The listing builds one solid part. Answer for the finished solid, in the listing's coordinates (mm). Face numbers are marked on the shaded views. A direction names the side the tool comes from. Round coordinates to 2 decimals unless told otherwise and drop trailing zeros. Write each loop counter-clockwise with the first axis right and the second up, starting at its lowest first coordinate (ties: lowest second). Pieces come first, ordered by that corner, then holes.
(1) For the marked faces 1 and 2, determine the directions among +Z, -Z, +X, -X, +Y, -Y from which every point of the face is accessible in a straight line to the end or side of a thin tool.
(2) The mould has two halves that part along Y. Classify the marked faces 3, 4, 5 and 6: +Y half, -Y half, draft (parallel to the pull), parting line (faces both ways), or undercut.
(3) Each of these flat-tipped pins is pushed along its axis until it touches: pin 1 Ø0.9 at (x, y) = (-99, 20) entering from -Z; pin 2 Ø3 at (y, z) = (4.5, 0.5) entering from -X; pin 3 Ø0.9 at (x, y) = (-97.5, 14.5) entering from +Z; pin 4 Ø5 at (y, z) = (17, 0.5) entering from -X. Where does it stop, or does it pass through?
(4) Find the intervals of material crossed by probe 1 along X at (y, z) = (14, -14); probe 2 along Y at (x, z) = (7, 15.5); probe 3 along Z at (x, y) = (6.5, 28), in increasing order.
(5) A cutting plane is placed at A-A, the plane z = 17.5. Give the vertices of the cut face in (x, y), and give its area (3 significant figures).
(6) A cutting plane is placed at C-C, the plane y = 6. Give the number of separate pieces and of enclosed holes in the cut face, and give its area (3 significant figures).
from build123d import *

# Parameters (mm, degrees)
SKETCH1_W           = 192
SKETCH1_H           = 42.3
BOSS_EXTRUDE1_DEPTH = 2
SKETCH2_W           = 176
SKETCH2_H           = 2
BOSS_EXTRUDE2_DEPTH = 30.35
SKETCH3_W           = 192
SKETCH3_H           = 42.3
BOSS_EXTRUDE3_DEPTH = 2
FILLET1_R           = 12
FILLET2_R           = 12
FILLET3_R           = 12
FILLET4_R           = 12
CUT_EXTRUDE1_DEPTH  = 2
CUT_EXTRUDE2_DEPTH  = 2
SKETCH6_R           = 4
BOSS_EXTRUDE5_DEPTH = 6
SKETCH7_R           = 2.25
CUT_EXTRUDE3_DEPTH  = 10
SKETCH8_W           = 1.5
SKETCH8_H           = 9.217326718
CUT_EXTRUDE4_DEPTH  = 6
SKETCH10_R          = 1.5
CUT_EXTRUDE9_DEPTH  = 6
FILLET5_R           = 2
FILLET6_R           = 2
FILLET9_R           = 2
FILLET10_R          = 2
FILLET11_R          = 2
FILLET14_R          = 1
FILLET15_R          = 1
SKETCH11_R          = 2.5
CUT_EXTRUDE11_DEPTH = 1
SKETCH12_R          = 4.5
CUT_EXTRUDE12_DEPTH = 1
SKETCH13_R          = 2.5
CUT_EXTRUDE14_DEPTH = 10
SKETCH14_W          = 29
SKETCH14_H          = 29
CUT_EXTRUDE15_DEPTH = 2
SKETCH15_R          = 4.5
CUT_EXTRUDE16_DEPTH = 1
FILLET16_R          = 0.5
FILLET17_R          = 0.5
SKETCH16_W          = 8
SKETCH16_H          = 30.35
CUT_EXTRUDE17_DEPTH = 80
FILLET18_R          = 2
FILLET19_R          = 2


with BuildPart() as part:
    # Sketch1 → Boss-Extrude1 (new body)
    with BuildSketch(Plane(origin=(0, 0, 0), x_dir=(1, 0, 0), z_dir=(0, 1, 0))):
        Rectangle(SKETCH1_W, SKETCH1_H)
    extrude(amount=BOSS_EXTRUDE1_DEPTH)

    # Sketch2 → Boss-Extrude2 (add)
    with BuildSketch(Plane(origin=(0, 2, 0), x_dir=(1, 0, 0), z_dir=(0, 1, 0))):
        Polygon((-96, 21.15), (-96, -21.15), (-88, -21.15), (-88, 19.15), (-88, 21.15), align=None)
        with Locations((0, 20.15)):
            Rectangle(SKETCH2_W, SKETCH2_H)
        Polygon((88, 19.15), (88, -21.15), (96, -21.15), (96, 21.15), (88, 21.15), align=None)
    extrude(amount=BOSS_EXTRUDE2_DEPTH)

    # Sketch3 → Boss-Extrude3 (add)
    with BuildSketch(Plane(origin=(0, 32.35, 0), x_dir=(1, 0, 0), z_dir=(0, 1, 0))):
        Rectangle(SKETCH3_W, SKETCH3_H)
    extrude(amount=BOSS_EXTRUDE3_DEPTH)

    # Fillet1
    fillet1_edges = [part.edges().sort_by_distance(p)[0] for p in [
        (-88, 32.35, 1),
    ]]
    fillet(fillet1_edges, radius=FILLET1_R)

    # Fillet2
    fillet2_edges = [part.edges().sort_by_distance(p)[0] for p in [
        (-88, 2, 1),
    ]]
    fillet(fillet2_edges, radius=FILLET2_R)

    # Fillet3
    fillet3_edges = [part.edges().sort_by_distance(p)[0] for p in [
        (88, 32.35, 1),
    ]]
    fillet(fillet3_edges, radius=FILLET3_R)

    # Fillet4
    fillet4_edges = [part.edges().sort_by_distance(p)[0] for p in [
        (88, 2, 1),
    ]]
    fillet(fillet4_edges, radius=FILLET4_R)

    # Sketch4 → Cut-Extrude1 (cut)
    with BuildSketch(Plane.XY.offset(-19.15)):
        with BuildLine():
            Line((-76, 32.35), (-88, 20.35))
            ThreePointArc((-88, 20.35), (-84.485281374, 28.835281374), (-76, 32.35))
        make_face()
        with BuildLine():
            Line((-88, 14), (-76, 2))
            ThreePointArc((-76, 2), (-84.485281374, 5.514718626), (-88, 14))
        make_face()
        Polygon((-76, 32.35), (-88, 20.35), (-88, 14), (-76, 2), (-26, 2), (-26, 32.35), align=None)
    extrude(amount=-CUT_EXTRUDE1_DEPTH, mode=Mode.SUBTRACT)

    # Sketch5 → Cut-Extrude2 (cut)
    with BuildSketch(Plane.XY.offset(-19.15)):
        Polygon((88, 20.35), (76, 32.35), (26, 32.35), (26, 2), (76, 2), (88, 14), align=None)
        with BuildLine():
            Line((88, 20.35), (76, 32.35))
            ThreePointArc((76, 32.35), (84.485281374, 28.835281374), (88, 20.35))
        make_face()
        with BuildLine():
            Line((76, 2), (88, 14))
            ThreePointArc((88, 14), (84.485281374, 5.514718626), (76, 2))
        make_face()
    extrude(amount=-CUT_EXTRUDE2_DEPTH, mode=Mode.SUBTRACT)

    # Sketch6 → Boss-Extrude5 (add)
    with BuildSketch(Plane.ZY.offset(96)):
        with Locations(Location((0, 17.175, 0), (0, 0, 180))):
            Circle(SKETCH6_R)
    extrude(amount=BOSS_EXTRUDE5_DEPTH)

    # Sketch7 → Cut-Extrude3 (cut)
    with BuildSketch(Plane.ZY.offset(102)):
        with Locations((0, 17.175)):
            Circle(SKETCH7_R)
    extrude(amount=-CUT_EXTRUDE3_DEPTH, mode=Mode.SUBTRACT)

    # Sketch8 → Cut-Extrude4 (cut)
    with BuildSketch(Plane.ZY.offset(102)):
        with Locations((0, 17.175)):
            Rectangle(SKETCH8_W, SKETCH8_H)
    extrude(amount=-CUT_EXTRUDE4_DEPTH, mode=Mode.SUBTRACT)

    # Sketch10 → Cut-Extrude9 (cut)
    with BuildSketch(Plane.XZ):
        with Locations(Location((-18.002866527, -3.655663128, 0), (0, 0, 270))):
            Circle(SKETCH10_R)
        with Locations(Location((17.997133473, -3.655663128, 0), (0, 0, 270))):
            Circle(SKETCH10_R)
    extrude(amount=-CUT_EXTRUDE9_DEPTH, mode=Mode.SUBTRACT)

    # Fillet5
    fillet5_edges = [part.edges().sort_by_distance(p)[0] for p in [
        (0, 0, -21.15),
    ]]
    fillet(fillet5_edges, radius=FILLET5_R - 0.0001)  # a hair under: the kernel refuses the full size

    # Fillet6
    fillet6_edges = [part.edges().sort_by_distance(p)[0] for p in [
        (0, 34.35, -21.15),
    ]]
    fillet(fillet6_edges, radius=FILLET6_R - 0.0001)  # a hair under: the kernel refuses the full size

    # Fillet9
    fillet9_edges = [part.edges().sort_by_distance(p)[0] for p in [
        (96, 0.585757148, -20.564242852),
        (96, 17.175, -21.15),
        (96, 33.764242852, -20.564242852),
        (96, 34.35, 0.99995),
        (96, 0, 0.99995),
    ]]
    fillet(fillet9_edges, radius=FILLET9_R - 0.0001)  # a hair under: the kernel refuses the full size

    # Fillet10
    fillet10_edges = [part.edges().sort_by_distance(p)[0] for p in [
        (-96, 0, 0.99995),
        (-96, 0.585757148, -20.564242852),
        (-96, 34.35, 0.99995),
        (-96, 17.175, -21.15),
        (-96, 33.764242852, -20.564242852),
    ]]
    fillet(fillet10_edges, radius=FILLET10_R - 0.0001)  # a hair under: the kernel refuses the full size

    # Fillet11
    fillet11_edges = [part.edges().sort_by_distance(p)[0] for p in [
        (96, 17.175, 21.15),
        (95.414242852, 0.585757148, 21.15),
        (95.414242852, 33.764242852, 21.15),
        (0, 34.35, 21.15),
        (-96, 17.175, 21.15),
        (0, 0, 21.15),
        (-95.414242852, 0.585757148, 21.15),
        (-95.414242852, 33.764242852, 21.15),
    ]]
    fillet(fillet11_edges, radius=FILLET11_R - 0.0001)  # a hair under: the kernel refuses the full size

    # Fillet14
    fillet14_edges = [part.edges().sort_by_distance(p)[0] for p in [
        (-102, 17.175, 4),
    ]]
    fillet(fillet14_edges, radius=FILLET14_R)

    # Fillet15
    fillet15_edges = [part.edges().sort_by_distance(p)[0] for p in [
        (-102, 17.175, -4),
    ]]
    fillet(fillet15_edges, radius=FILLET15_R)

    # Sketch11 → Cut-Extrude11 (cut)
    with BuildSketch(Plane(origin=(0, 0, 0), x_dir=(-1, 0, 0), z_dir=(0, -1, 0))):
        with Locations(Location((18.002866527, 3.655663128, 0), (0, 0, 90))):
            Circle(SKETCH11_R)
        with Locations(Location((-17.997133473, 3.655663128, 0), (0, 0, 90))):
            Circle(SKETCH11_R)
    extrude(amount=-CUT_EXTRUDE11_DEPTH, mode=Mode.SUBTRACT)

    # Sketch12 → Cut-Extrude12 (cut)
    with BuildSketch(Plane(origin=(96, 0, 0), x_dir=(0, 0, -1), z_dir=(1, 0, 0))):
        with Locations((0.090844805, 17.432374702)):
            Circle(SKETCH12_R)
    extrude(amount=-CUT_EXTRUDE12_DEPTH, mode=Mode.SUBTRACT)

    # Sketch13 → Cut-Extrude14 (cut)
    with BuildSketch(Plane(origin=(96, 0, 0), x_dir=(0, 0, -1), z_dir=(1, 0, 0))):
        with Locations((0.090844805, 17.432374702)):
            Circle(SKETCH13_R)
    extrude(amount=-CUT_EXTRUDE14_DEPTH, mode=Mode.SUBTRACT)

    # Sketch14 → Cut-Extrude15 (cut)
    with BuildSketch(Plane(origin=(96, 0, 0), x_dir=(0, 0, -1), z_dir=(1, 0, 0))):
        with Locations((0.090844805, 17.432374702)):
            Rectangle(SKETCH14_W, SKETCH14_H)
    extrude(amount=-CUT_EXTRUDE15_DEPTH, mode=Mode.SUBTRACT)

    # Sketch15 → Cut-Extrude16 (cut)
    with BuildSketch(Plane(origin=(94, 0, 0), x_dir=(0, 0, -1), z_dir=(1, 0, 0))):
        with Locations((0.090844805, 17.432374702)):
            Circle(SKETCH15_R)
    extrude(amount=-CUT_EXTRUDE16_DEPTH, mode=Mode.SUBTRACT)

    # Fillet16
    fillet16_edges = [part.edges().sort_by_distance(p)[0] for p in [
        (-102, 18.474038106, 1.837117307),
    ]]
    fillet(fillet16_edges, radius=FILLET16_R)

    # Fillet17
    fillet17_edges = [part.edges().sort_by_distance(p)[0] for p in [
        (-102, 17.175, -2.25),
    ]]
    fillet(fillet17_edges, radius=FILLET17_R)

    # Sketch16 → Cut-Extrude17 (cut)
    with BuildSketch(Plane(origin=(0, 0, -21.15), x_dir=(-1, 0, 0), z_dir=(0, 0, -1))):
        with Locations((-22, 17.175)):
            Rectangle(SKETCH16_W, SKETCH16_H)
        with Locations((22, 17.175)):
            Rectangle(SKETCH16_W, SKETCH16_H)
    extrude(amount=-CUT_EXTRUDE17_DEPTH, mode=Mode.SUBTRACT)

    # Fillet18
    fillet18_edges = [part.edges().sort_by_distance(p)[0] for p in [
        (-18, 17.175, -21.15),
    ]]
    fillet(fillet18_edges, radius=FILLET18_R - 0.0001)  # a hair under: the kernel refuses the full size

    # Fillet19
    fillet19_edges = [part.edges().sort_by_distance(p)[0] for p in [
        (18, 17.175, -21.15),
    ]]
    fillet(fillet19_edges, radius=FILLET19_R - 0.0001)  # a hair under: the kernel refuses the full size


solid = part.part
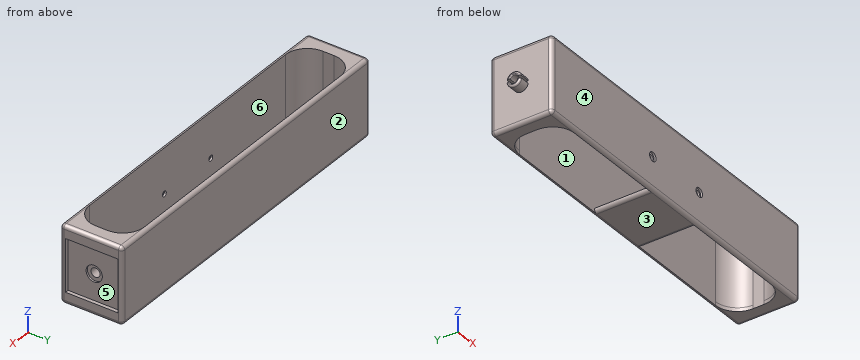
Solutions:
1. face 1: +Z
1. face 2: +Z, -Z, +X, -X, +Y
2. face 3: draft
2. face 4: -Y half
2. face 5: undercut
2. face 6: undercut
3. pin 1: stops at z = -3.22
3. pin 2: stops at x = -96
3. pin 3: stops at z = 3.32
3. pin 4: stops at x = -102
4. probe 1: x = -96 to -88, 88 to 94
4. probe 2: y = 0 to 2, 32.35 to 34.35
4. probe 3: z = -21.15 to -19.15
5. outline: (-96, 2) arc R2 ccw to (-94, 0) - (94, 0) arc R2 ccw to (96, 2) - (96, 32.35) arc R2 ccw to (94, 34.35) - (-94, 34.35) arc R2 ccw to (-96, 32.35) - close; hole (-88, 14) arc R12 ccw to (-76, 2) - (76, 2) arc R12 ccw to (88, 14) - (88, 20.35) arc R12 ccw to (76, 32.35) - (-76, 32.35) arc R12 ccw to (-88, 20.35) - close
5. area: 1,370 mm2
6. separate pieces: 3
6. enclosed holes: 0
6. area: 944 mm2
